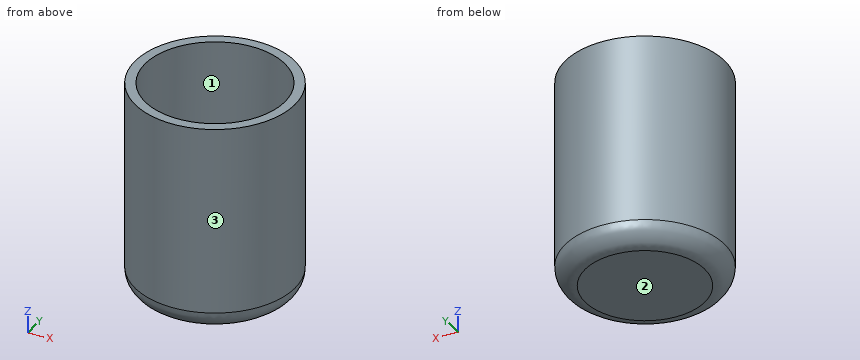
from build123d import *

# Parameters (mm, degrees)
F0_R     = 40
F0_R_2   = 35
F0_R_3   = 30
F1_DEPTH = 50
F2_DEPTH = 100
F3_DEPTH = 5
F4_R     = 10


with BuildPart() as f1:
    # F0 (on Top) → F1 (new body)
    with BuildSketch(Plane.XY):
        Circle(F0_R)
        Circle(F0_R_2, mode=Mode.SUBTRACT)
        Circle(F0_R_2)
        Circle(F0_R_3, mode=Mode.SUBTRACT)
    extrude(amount=F1_DEPTH)

    # F0 (on Top) → F2 (join)
    with BuildSketch(Plane.XY):
        Circle(F0_R)
        Circle(F0_R_2, mode=Mode.SUBTRACT)
    extrude(amount=F2_DEPTH)

    # F0 (on Top) → F3 (join)
    with BuildSketch(Plane.XY):
        Circle(F0_R)
        Circle(F0_R_2, mode=Mode.SUBTRACT)
        Circle(F0_R_2)
        Circle(F0_R_3, mode=Mode.SUBTRACT)
        Circle(F0_R_3)
    extrude(amount=-F3_DEPTH)

    # F4
    f4_edges = [f1.edges().sort_by_distance(p)[0] for p in [
        (-40, 0, -5),
    ]]
    fillet(f4_edges, radius=F4_R)


solid = f1.part
The listing builds one solid part. Answer for the finished solid, in the listing's coordinates (mm). Face numbers are marked on the shaded views. Round coordinates to 2 decimals unless told otherwise and drop trailing zeros. Order: outer loops, then holes, each group sorted by start corner. A loop starts at its lowest first (then second) coordinate and runs counter-clockwise, first axis right, second up. Notation, with made-up numbers: (15.5, -10) -> (46.5, -10) arc R5 ccw to (46.5, -4) -> close; hole circle Ø9 at (49, -19.75). An arc over 180 degrees is marked (long way). One line per item, written item: value.
Item 1: Find section A-A, the plane z = 70. Give the vertices of the cut face in (x, y), then the cut area to 3 significant figures.
Taken from the geometry:
outline: circle Ø80 at (0, 0); hole circle Ø70 at (0, 0)
area: 1,180 mm2
Item 2: Straight lines are drawn through the part: L1, parallel to Y at x = 0, z = 23.5; L2, parallel to X at y = 0, z = 80.5; L3, parallel to Z at x = 6.5, y = 24.5. For each, find the intervals that lie inside material, in ascending order.
Taken from the geometry:
L1: y = -40 to -30, 30 to 40
L2: x = -40 to -35, 35 to 40
L3: z = -5 to 0
Item 3: Find section B-B, the plane z = 29.5. Give the vertices of the cut face in (x, y).
Taken from the geometry:
outline: circle Ø80 at (0, 0); hole circle Ø60 at (0, 0)
Item 4: Given P1, Ø12, axis at y = 29, z = 45, coming from the -X side; P2, Ø1.5, axis at x = -30.5, y = 25, coming from the -Z side; P3, Ø10, axis at y = 24, z = 38, coming from the -X side, each flat-ended and moving along its own axis, determine where each tip first touches the part or whether it passes through.
Taken from the geometry:
P1: stops at x = -32.73
P2: stops at z = 0.05
P3: stops at x = -35.2
Item 5: For a pull along X with two mould halves and no side action, classify the marked faces 1, 2 and 3 as released by +X, released by -X, zero draft, split by the parting line, or undercut.
Taken from the geometry:
face 1: undercut
face 2: zero draft
face 3: split by the parting line
